```python
from build123d import *

# Parameters (mm, degrees)
SKETCH1_W           = 20
SKETCH1_H           = 20
BOSS_EXTRUDE1_DEPTH = 20
SKETCH3_R           = 2.5
CUT_EXTRUDE1_DEPTH  = 35.641016151
SKETCH4_R           = 2.5
CUT_EXTRUDE2_DEPTH  = 15


with BuildPart() as part:
    # Sketch1 → Boss-Extrude1 (new body)
    with BuildSketch(Plane(origin=(0, 0, 0), x_dir=(1, 0, 0), z_dir=(0, 1, 0))):
        with Locations((-10, 10)):
            Rectangle(SKETCH1_W, SKETCH1_H)
    extrude(amount=BOSS_EXTRUDE1_DEPTH)

    # Sketch3 → Cut-Extrude1 (cut, through all)
    with BuildSketch(Plane(origin=(0, 0, 0), x_dir=(0, 0, -1), z_dir=(1, 0, 0))):
        with Locations((10, 15.5)):
            Circle(SKETCH3_R)
    extrude(amount=-CUT_EXTRUDE1_DEPTH, mode=Mode.SUBTRACT)

    # Sketch4 → Cut-Extrude2 (cut)
    with BuildSketch(Plane(origin=(0, 0, 0), x_dir=(0, 0, -1), z_dir=(1, 0, 0))):
        with Locations((10, 9.5)):
            Circle(SKETCH4_R)
    extrude(amount=-CUT_EXTRUDE2_DEPTH, mode=Mode.SUBTRACT)


solid = part.part
```
Could you check a few things on this model? Use its own coordinates, in mm. A direction names the side the tool comes from. Round coordinates to 2 decimals unless told otherwise and drop trailing zeros. Loops run counter-clockwise (first coordinate to the right, second up) from the corner with the lowest first, then second, coordinate; pieces in that order, holes last.
Q1. Please list where these lines run through material, in increasing order: L1, parallel to Y at x = -12.75, z = -10; L2, parallel to Z at x = -3, y = 17.5; L3, parallel to Z at x = -12.75, y = 7.25.
Q2. I want a section at B-B (z = -12). Write out the boundary of the cut face in (x, y).
Q3. I want a section at D-D (z = -10). Write out the boundary of the cut face in (x, y), and give its area (3 significant figures).
Q4. Thinking about a two-plate mould opening in Z: for faces 3 (the flat face through (-10, 10, -20)), 4 (the cylindrical face through (-9.86, 13.06, -9.46)), 5 (the flat face through (-20, 10, -10)), which applies, pulls with the +Z half, pulls with the -Z half, needs draft (parallel to the pull), parting line crosses it, or undercut?
Q5. For P1, Ø12, axis at x = -9.5, y = 12, coming from the +Z side; P2, Ø4, axis at y = 15.5, z = -10, coming from the -X side; P3, Ø4.5, axis at y = 9.5, z = -10, coming from the +X side, each with a flat end and sliding along its axis, tell me the tip position at first contact or that it passes through.
Q6. I want a section at C-C (x = -5.5). Write out the boundary of the cut face in (y, z), and give its area (3 significant figures).
Q7. I want a section at A-A (y = 15.5). Write out the boundary of the cut face in (x, z).
Q8. On a 3-axis mill with a long thin cutter (end or side, diameter ignored), from which of +Z, -Z, +X, -X, +Y, -Y can I reach the whole of each face in a straight line? I mean faces 1 (the flat face through (-10, 10, 0)), 2 (the flat face through (-15, 10, -10)). Say none if no direction works.
Answer below:
1. L1: y = 0 to 7, 12 to 13, 18 to 20
1. L2: z = -20 to -11.5, -8.5 to 0
1. L3: z = -20 to -11.09, -8.91 to 0
2. outline: (-20, 0) - (0, 0) - (0, 8) - (-15, 8) - (-15, 11) - (0, 11) - (0, 14) - (-20, 14) - close; (-20, 17) - (0, 17) - (0, 20) - (-20, 20) - close
3. outline: (-20, 0) - (0, 0) - (0, 7) - (-15, 7) - (-15, 12) - (0, 12) - (0, 13) - (-20, 13) - close; (-20, 18) - (0, 18) - (0, 20) - (-20, 20) - close
3. area: 225 mm2
4. face 3: pulls with the -Z half
4. face 4: undercut
4. face 5: needs draft
5. P1: stops at z = 0
5. P2: passes through
5. P3: stops at x = -15
6. outline: (0, -20) - (20, -20) - (20, 0) - (0, 0) - close; hole circle Ø5 at (9.5, -10); hole circle Ø5 at (15.5, -10)
6. area: 361 mm2
7. outline: (-20, -20) - (0, -20) - (0, -12.5) - (-20, -12.5) - close; (-20, -7.5) - (0, -7.5) - (0, 0) - (-20, 0) - close
8. face 1: +Z, +X, -X, +Y, -Y
8. face 2: +X
